Read the model definition and answer for the solid it produces. Units are mm, in the model's axes. A direction names the side the tool comes from. Round coordinates to 2 decimals unless told otherwise and drop trailing zeros. Order: outer loops, then holes, each group sorted by start corner. A loop starts at its lowest first (then second) coordinate and runs counter-clockwise, first axis right, second up. Notation, with made-up numbers: (58.5, -25.5) - (90.5, -25.5) arc R18 cw to (90.5, -15.5) - close; hole circle Ø2 at (27.25, -1.75). An arc over 180 degrees is marked (long way). Answer as a JSON object with one key per item and string values. Group by question number.
Q1. The mould has two halves that part along X. Classify faces 4 (the cylindrical face through (20.765, -39.923, 0.966)), 5 (the conical face through (-0.013, 40.286, -53.181)), 6 (the flat face through (23.1, -26.5, -69)): pulls with the +X half, pulls with the -X half, needs draft (parallel to the pull), parting line crosses it, or undercut.
Q2. A cutting plane is placed at A-A on y = 0. Determine the outline of the cut face in (x, z).
Q3. A cutting plane is placed at C-C on y = 10. Determine the outline of the cut face in (x, z).
Q4. Given pin 1 Ø8 at (x, z) = (-17, 50.5) entering from -Y; pin 2 Ø3 at (x, z) = (34.5, 33.5) entering from -Y; pin 3 Ø2.5 at (x, y) = (-34.64, -20) entering from +Z; pin 4 Ø6 at (x, y) = (-31.5, 1.5) entering from -Z, each flat-ended and moving along its own axis, determine where each tip first touches the part or whether it passes through.
Q5. A tool of negligible diameter and unlimited length cuts with its end or side. For faces 1 (the cylindrical face through (20.2, 33.24, 28.93)), 2 (the cylindrical face through (-0.07, 41.65, -61.6)), 3 (the cylindrical face through (-0.07, 41.65, 61.6)), from which of +Z, -Z, +X, -X, +Y, -Y can it reach the whole face along a straight path? Write none if from no direction.
Q6. A cutting plane is placed at B-B on z = -50. Determine the outline of the cut face in (x, y), and give its area (3 significant figures).
Q7. A cutting plane is placed at D-D on z = -2. Determine the outline of the cut face in (x, y), and give its area (3 significant figures).
Q8. Consider line 1 (Y direction, x = 0, z = -63); line 2 (X direction, y = -20, z = -60); line 3 (Y direction, x = 0, z = -2). Determine where each line is inside the solid, lowest interval first.
```python
from build123d import *

# Parameters (mm, degrees)
CROQUIS1_R                     = 45
CROQUIS1_R_2                   = 35
SALIENTE_EXTRUIR1_DEPTH        = 69
CORTAR_EXTRUIR1_DEPTH          = 138
CROQUIS3_R                     = 37.5
CORTAR_EXTRUIR2_DEPTH          = 138
TALADRO_ROSCADO_M41_AT_2_COUNT = 2
TALADRO_ROSCADO_M41_AT_2_PITCH = 69.282032303
TALADRO_ROSCADO_M41_AT_3_COUNT = 2
TALADRO_ROSCADO_M41_AT_3_PITCH = 69.282032303


with BuildPart() as part:
    # Croquis1 → Saliente-Extruir1 (new body, symmetric)
    with BuildSketch(Plane.XY):
        Circle(CROQUIS1_R)
        Circle(CROQUIS1_R_2, mode=Mode.SUBTRACT)
    extrude(amount=SALIENTE_EXTRUIR1_DEPTH, both=True)

    # Croquis2 → Cortar-Extruir1 (cut)
    with BuildSketch(Plane(origin=(0, 0, 0), x_dir=(1, 0, 0), z_dir=(0, 1, 0))):
        with BuildLine():
            Line((-26.3, 43), (18.7, 43))
            Line((18.7, 43), (18.7, 32.5))
            ThreePointArc((18.7, 32.5), (20.164466094, 28.964466094), (23.7, 27.5))
            Line((23.7, 27.5), (26.7, 27.5))
            Line((26.7, 27.5), (26.7, -27.5))
            Line((26.7, -27.5), (23.7, -27.5))
            ThreePointArc((23.7, -27.5), (20.164466094, -28.964466094), (18.7, -32.5))
            Line((18.7, -32.5), (18.7, -42.7))
            Line((18.7, -42.7), (-26.3, -42.7))
            Line((-26.3, -42.7), (-26.3, 43))
        make_face()
    extrude(amount=CORTAR_EXTRUIR1_DEPTH, mode=Mode.SUBTRACT)

    # Croquis3 → Cortar-Extruir2 (cut)
    with BuildSketch(Plane(origin=(0, 0, 0), x_dir=(0, 0, -1), z_dir=(1, 0, 0))):
        with Locations((0, 59)):
            Circle(CROQUIS3_R)
    extrude(amount=-CORTAR_EXTRUIR2_DEPTH, mode=Mode.SUBTRACT)

    # Croquis5 → Taladro roscado M41 (revolve, cut)
    with BuildSketch(Plane(origin=(0, 40, 69), x_dir=(0, -1, 0), z_dir=(1, 0, 0))):
        Polygon((0, 0), (0, 15.991420021), (1.65, 15), (1.65, 0), align=None)
    taladro_roscado_m41 = revolve(axis=Axis((0, 40, 75.35), (0, 0, -1)), mode=Mode.SUBTRACT)

    # Taladro roscado M41 at 2: Taladro roscado M41 ×2
    with Locations(*[Vector(0.5, -0.866025404, 0) * (i * TALADRO_ROSCADO_M41_AT_2_PITCH) for i in range(1, TALADRO_ROSCADO_M41_AT_2_COUNT)]):
        add(taladro_roscado_m41, mode=Mode.SUBTRACT)

    # Taladro roscado M41 at 3: Taladro roscado M41 ×2
    with Locations(*[Vector(-0.5, -0.866025404, 0) * (i * TALADRO_ROSCADO_M41_AT_3_PITCH) for i in range(1, TALADRO_ROSCADO_M41_AT_3_COUNT)]):
        add(taladro_roscado_m41, mode=Mode.SUBTRACT)

    # Simetría1: Taladro roscado M41 across plane
    add(taladro_roscado_m41.mirror(Plane.XY), mode=Mode.SUBTRACT)

    # Simetría1 copy 1 sketch → Simetría1 copy 1 (revolve, cut)
    with BuildSketch(Plane(origin=(34.641016151, -20, -69), x_dir=(0, -1, 0), z_dir=(1, 0, 0))):
        Polygon((0, 0), (0, -15.991420021), (1.65, -15), (1.65, 0), align=None)
    revolve(axis=Axis((34.641016151, -20, -75.35), (0, 0, -1)), mode=Mode.SUBTRACT)

    # Simetría1 copy 2 sketch → Simetría1 copy 2 (revolve, cut)
    with BuildSketch(Plane(origin=(-34.641016151, -20, -69), x_dir=(0, -1, 0), z_dir=(1, 0, 0))):
        Polygon((0, 0), (0, -15.991420021), (1.65, -15), (1.65, 0), align=None)
    revolve(axis=Axis((-34.641016151, -20, -75.35), (0, 0, -1)), mode=Mode.SUBTRACT)


solid = part.part
```
Result set:
{
 "1": {"face 4": "parting line crosses it", "face 5": "undercut", "face 6": "needs draft"},
 "2": {"outline": "(-45, -69) - (-35, -69) - (-35, 69) - (-45, 69) - close; (35, -69) - (45, -69) - (45, 69) - (35, 69) - close"},
 "3": {"outline": "(-43.87, -69) - (-33.54, -69) - (-33.54, 69) - (-43.87, 69) - close; (33.54, -69) - (43.87, -69) - (43.87, 69) - (33.54, 69) - close"},
 "4": {"pin 1": "stops at y = -43.08", "pin 2": "stops at y = -30.59", "pin 3": "stops at z = 53.76", "pin 4": "passes through"},
 "5": {"face 1": "+Y", "face 2": "-Z", "face 3": "+Z"},
 "6": {"outline": "circle Ø90 at (0, 0); hole circle Ø70 at (0, 0)", "area": "2,510 mm²"},
 "7": {"outline": "(-39.5, 21.55) arc R45 ccw (long way) to (26.7, 36.22) - (26.7, 22.63) arc R35 cw (long way) to (-27.58, 21.55) - close", "area": "1,820 mm²"},
 "8": {"line 1": "y = -45 to -35, 35 to 38.35, 41.65 to 45", "line 2": "x = -40.31 to -36.29, -32.99 to -28.72, 28.72 to 32.99, 36.29 to 40.31", "line 3": "y = -45 to -35"}
}
